For this review, take the finished solid that the model builds, in its own axes (mm). A direction names the side the tool comes from. Coordinates: 2 decimals unless noted, no trailing zeros. Write each loop counter-clockwise with the first axis right and the second up, starting at its lowest first coordinate (ties: lowest second). Pieces come first, ordered by that corner, then holes.
```python
from build123d import *

# Parameters (mm, degrees)
SWEEP1_START   = -13.5
SWEEP1_DEPTH   = 10
SWEEP1_START_2 = 3.5
SWEEP1_2_DEPTH = 10
SWEEP1_START_3 = -3.5
SWEEP1_3_DEPTH = 7
SKETCH12_R     = 1


# Read off the part's stored shape, not the designer's step: Sweep1
with BuildPart() as part:
    # Sweep1 outline → Sweep1 (new body)
    with BuildSketch(Plane.XY.offset(SWEEP1_START)):
        Polygon((-7.642649587, 204.357350413), (-7.642649587, 220), (-12, 220), (-12, 200), (0, 200), (0, 0), (-200, 0), (-200, 12), (-220, 12), (-220, 7.642649587), (-204.357350413, 7.642649587), (-204.357350413, -4.357350413), (4.357350413, -4.357350413), (4.357350413, 204.357350413), align=None)
    extrude(amount=SWEEP1_DEPTH)



with BuildPart() as body_2:
    # Sweep1 2 outline → Sweep1 2 (new body)
    with BuildSketch(Plane.XY.offset(SWEEP1_START_2)):
        Polygon((-7.642649587, 204.357350413), (-7.642649587, 220), (-12, 220), (-12, 200), (0, 200), (0, 0), (-200, 0), (-200, 12), (-220, 12), (-220, 7.642649587), (-204.357350413, 7.642649587), (-204.357350413, -4.357350413), (4.357350413, -4.357350413), (4.357350413, 204.357350413), align=None)
    extrude(amount=SWEEP1_2_DEPTH)


with BuildPart() as part_1:
    add(part.part)

    add(body_2.part)  # Sweep1 3 merges body 2
    # Sweep1 3 outline → Sweep1 3 (add)
    with BuildSketch(Plane.XY.offset(SWEEP1_START_3)):
        Polygon((-11.392649587, 200.607350413), (-11.392649587, 220), (-15.74831078, 220), (-15.74831078, 196.25168922), (-3.74831078, 196.25168922), (-3.74831078, 3.74831078), (-196.25168922, 3.74831078), (-196.25168922, 15.74831078), (-220, 15.74831078), (-220, 11.392649587), (-200.607350413, 11.392649587), (-200.607350413, -0.607350413), (0.607350413, -0.607350413), (0.607350413, 200.607350413), align=None)
    extrude(amount=SWEEP1_3_DEPTH)

    # Sweep2: sweep along a path in Sketch11
    with BuildLine(Plane.XY) as sweep2_path:
        Line((-30, 0), (0, 30))
    # Sketch12 → Sweep2 (sweep)
    with BuildSketch(Plane(origin=(0, 0, 0), x_dir=(0, 0, -1), z_dir=(1, 0, 0))):
        with Locations((0, 30)):
            Circle(SKETCH12_R)
    sweep(path=sweep2_path.line)


solid = part_1.part
```
Q1. Add section A-A (x = -72). State the section outline as (y, z) points, then the cut area to 3 significant figures.
Ans:
outline: (-4.36, -13.5) - (0, -13.5) - (0, -3.5) - (3.75, -3.5) - (3.75, 3.5) - (0, 3.5) - (0, 13.5) - (-4.36, 13.5) - (-4.36, 3.5) - (-0.61, 3.5) - (-0.61, -3.5) - (-4.36, -3.5) - close
area: 118 mm2
Q2. Add section C-C (y = 123). State the section outline as (x, z) points, then the cut area to 3 significant figures.
Ans:
outline: (-3.75, -3.5) - (0, -3.5) - (0, -13.5) - (4.36, -13.5) - (4.36, -3.5) - (0.61, -3.5) - (0.61, 3.5) - (4.36, 3.5) - (4.36, 13.5) - (0, 13.5) - (0, 3.5) - (-3.75, 3.5) - close
area: 118 mm2
Q3. Draft analysis for pull direction X (two halves, no side actions). For faces 5 (the flat face through (-208, 15.748, 0)), 6 (the flat face through (-200, 6, -9)), 7 (the flat face through (-7.643, 212, 8)), state which applies: +X half, -X half, draft (parallel to the pull), parting line (faces both ways), or undercut.
Ans:
face 5: draft
face 6: undercut
face 7: +X half
Q4. Clearance check with flat-ended pins moving along their axes: pin 1 Ø3 at (x, z) = (-210.5, 11) entering from +Y; pin 2 Ø2 at (y, z) = (105.5, 0.5) entering from +X; pin 3 Ø5 at (x, z) = (-99.5, 8) entering from +Y. State where each tip first meets the part, or that it passes through.
Ans:
pin 1: stops at y = 12
pin 2: stops at x = 0.61
pin 3: stops at y = 0
Q5. Tool access review of faces 1 (the flat face through (-10, 196.252, 0)), 2 (the flat face through (-5, 200.607, 0)), 3 (the flat face through (-204.357, 2, 8)), 4 (the flat face through (-6, 200, 8)): name each direction out of +Z, -Z, +X, -X, +Y, -Y from which nothing blocks a thin tool from reaching the whole face with its end or side.
Ans:
face 1: +Z, -Z, -X
face 2: +X, +Y
face 3: +Z, -Z, -X, -Y
face 4: +Z, -X
Q6. Add section B-B (z = -9.25). State the section outline as (x, y) points, then the cut area to 3 significant figures.
Ans:
outline: (-220, 7.64) - (-204.36, 7.64) - (-204.36, -4.36) - (4.36, -4.36) - (4.36, 204.36) - (-7.64, 204.36) - (-7.64, 220) - (-12, 220) - (-12, 200) - (0, 200) - (0, 0) - (-200, 0) - (-200, 12) - (-220, 12) - close
area: 2,040 mm2
Q7. For probe 1 along Y at (x, z) = (-198.5, 8); probe 2 along Y at (x, z) = (-159, 1.25); probe 3 along X at (y, z) = (165, -8.5), list the stretches that pass through material, from the lowest coordinate up.
Ans:
probe 1: y = -4.36 to 0
probe 2: y = -0.61 to 3.75
probe 3: x = 0 to 4.36
